from build123d import *

# Parameters (mm, degrees)
SKETCH1_R           = 2.9337
BOSS_EXTRUDE1_DEPTH = 50.8


with BuildPart() as part:
    # Sketch1 → Boss-Extrude1 (new body)
    with BuildSketch(Plane(origin=(0, 0, 0), x_dir=(-1, 0, 0), z_dir=(0, 0, -1))):
        with BuildLine():
            Line((-4.70551159, -4.549815043), (-3.666174521, -6.349999904))
            Line((-3.666174521, -6.349999904), (-1.587500385, -6.349999904))
            ThreePointArc((-1.587500385, -6.349999904), (-3.85e-07, -4.762499904), (1.587499615, -6.349999904))
            Line((1.587499615, -6.349999904), (3.666173825, -6.349999904))
            Line((3.666173825, -6.349999904), (4.705510942, -4.54981524))
            ThreePointArc((4.705510942, -4.54981524), (4.124445629, -2.381249907), (6.293010962, -1.800184594))
            Line((6.293010962, -1.800184594), (7.332348079, 7e-08))
            Line((7.332348079, 7e-08), (6.293011217, 1.800184685))
            ThreePointArc((6.293011217, 1.800184685), (4.124445939, 2.381250203), (4.705511457, 4.549815481))
            Line((4.705511457, 4.549815481), (3.666174521, 6.350000222))
            Line((3.666174521, 6.350000222), (1.587500385, 6.350000222))
            ThreePointArc((1.587500385, 6.350000222), (3.85e-07, 4.762500222), (-1.587499615, 6.350000222))
            Line((-1.587499615, 6.350000222), (-3.666173825, 6.350000222))
            Line((-3.666173825, 6.350000222), (-4.705511038, 4.549815614))
            ThreePointArc((-4.705511038, 4.549815614), (-4.124445841, 2.38125025), (-6.293011205, 1.800185053))
            Line((-6.293011205, 1.800185053), (-7.332348419, 4.44e-07))
            Line((-7.332348419, 4.44e-07), (-6.293011423, -1.80018429))
            ThreePointArc((-6.293011423, -1.80018429), (-4.12444613, -2.38124975), (-4.70551159, -4.549815043))
        make_face()
        Circle(SKETCH1_R, mode=Mode.SUBTRACT)
    extrude(amount=BOSS_EXTRUDE1_DEPTH)


solid = part.part
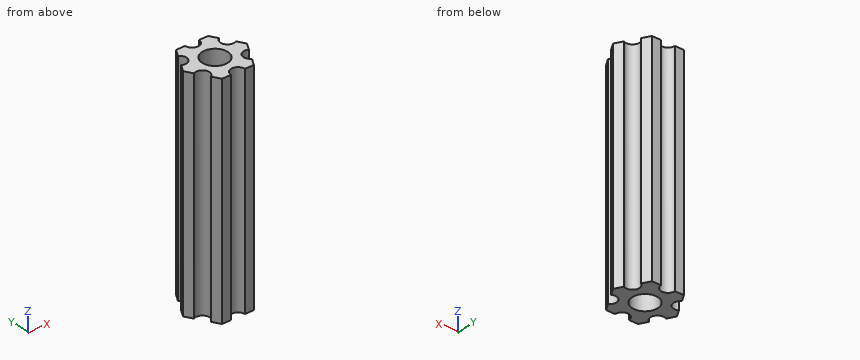
CAD build for the part. Positions are in the model's coordinates, mm. Coordinates: 2 decimals unless noted, no trailing zeros. Loops run counter-clockwise (first coordinate to the right, second up) from the corner with the lowest first, then second, coordinate; pieces in that order, holes last. Notation, with made-up numbers: (-0.75, 43) -> (13.25, 43) arc R15 cw to (13.25, 66) -> close; hole circle Ø1 at (42.5, 82.25). An arc over 180 degrees is marked (long way). One line per item, written item: value.
1. Drill centre lines: line 1 (Y direction, x = 0, z = -32); line 2 (X direction, y = 0.75, z = -32); line 3 (X direction, y = 0.5, z = -44). Where is each one in solid material? Low to high. Write a range as [from, to].
Answers:
line 1: y = [-4.76, -2.93], [2.93, 4.76]
line 2: x = [-6.9, -2.84], [2.84, 6.9]
line 3: x = [-7.04, -2.89], [2.89, 7.04]
2. Flat gauge pins, fed straight in: P1, Ø1, axis at y = -3.5, z = -31.5, coming from the +X side; P2, Ø2, axis at y = -0.5, z = -26, coming from the +X side; P3, Ø1.5, axis at y = 3.5, z = -12, coming from the +X side. Where does each tip first touch, or does it go through?
Answers:
P1: stops at x = 4.14
P2: stops at x = 7.33
P3: stops at x = 4.33
3. Slice it at B-B on x = 0. Write the cut outline in (y, z).
Answers:
outline: (-4.76, -50.8) -> (-2.93, -50.8) -> (-2.93, 0) -> (-4.76, 0) -> close; (2.93, -50.8) -> (4.76, -50.8) -> (4.76, 0) -> (2.93, 0) -> close
4. Slice it at C-C on y = 5.75. Write the cut outline in (x, z).
Answers:
outline: (-4.01, -50.8) -> (-1.47, -50.8) -> (-1.47, 0) -> (-4.01, 0) -> close; (1.47, -50.8) -> (4.01, -50.8) -> (4.01, 0) -> (1.47, 0) -> close
5. Slice it at D-D on x = 5.25. Write the cut outline in (y, z).
Answers:
outline: (-1.61, -50.8) -> (1.61, -50.8) -> (1.61, 0) -> (-1.61, 0) -> close
